from build123d import *

# Parameters (mm, degrees)
EXTRUDE_1_DEPTH     = 11
CUT_EXTRUDE_1_REACH = 15.892
SKETCH_2_R          = 1
CUT_EXTRUDE_2_REACH = 15.892
SKETCH_3_R          = 1


with BuildPart() as part:
    # 草图1 → 凸台-拉伸1 (new, symmetric)
    with BuildSketch(Plane(origin=(0, 0, 0), x_dir=(0, 0, -1), z_dir=(1, 0, 0))):
        Polygon((0, 0), (0, 6), (2, 6), (2, 2), (6, 2), (6, 0), align=None)
    extrude(amount=EXTRUDE_1_DEPTH, both=True)

    # 草图2 → 切除-拉伸1 (cut, up to next)
    with BuildSketch(Plane.XY, mode=Mode.PRIVATE) as cut_extrude_1_sk1:
        with Locations((-8.5, 4)):
            Circle(SKETCH_2_R)
    cut_extrude_1_tool1 = extrude(cut_extrude_1_sk1.sketch, amount=-CUT_EXTRUDE_1_REACH, mode=Mode.PRIVATE) & part.part
    # 草图2 → 切除-拉伸1 (cut, up to next)
    with BuildSketch(Plane.XY, mode=Mode.PRIVATE) as cut_extrude_1_sk2:
        with Locations((8.5, 4)):
            Circle(SKETCH_2_R)
    cut_extrude_1_tool2 = extrude(cut_extrude_1_sk2.sketch, amount=-CUT_EXTRUDE_1_REACH, mode=Mode.PRIVATE) & part.part
    add(cut_extrude_1_tool1.solids().sort_by_distance((-8.5, 4, 0))[0], mode=Mode.SUBTRACT)
    add(cut_extrude_1_tool2.solids().sort_by_distance((8.5, 4, 0))[0], mode=Mode.SUBTRACT)

    # 草图3 → 切除-拉伸2 (cut, up to next)
    with BuildSketch(Plane.XZ, mode=Mode.PRIVATE) as cut_extrude_2_sk1:
        with Locations(Location((-8.5, -4, 0), (0, 0, 270))):
            Circle(SKETCH_3_R)
    cut_extrude_2_tool1 = extrude(cut_extrude_2_sk1.sketch, amount=-CUT_EXTRUDE_2_REACH, mode=Mode.PRIVATE) & part.part
    # 草图3 → 切除-拉伸2 (cut, up to next)
    with BuildSketch(Plane.XZ, mode=Mode.PRIVATE) as cut_extrude_2_sk2:
        with Locations(Location((8.5, -4, 0), (0, 0, 270))):
            Circle(SKETCH_3_R)
    cut_extrude_2_tool2 = extrude(cut_extrude_2_sk2.sketch, amount=-CUT_EXTRUDE_2_REACH, mode=Mode.PRIVATE) & part.part
    add(cut_extrude_2_tool1.solids().sort_by_distance((-8.5, 0, -4))[0], mode=Mode.SUBTRACT)
    add(cut_extrude_2_tool2.solids().sort_by_distance((8.5, 0, -4))[0], mode=Mode.SUBTRACT)


solid = part.part
Build history of the part. All positions in model axes, mm. A direction names the side the tool comes from. Coordinates: 2 decimals unless noted, no trailing zeros. Order: outer loops, then holes, each group sorted by start corner. A loop starts at its lowest first (then second) coordinate and runs counter-clockwise, first axis right, second up. Notation, with made-up numbers: M 61.25,9 L 100.25,9 A22 cw 100.25,27 Z; hole C -18,75 d4. An arc over 180 degrees is marked long. One line per question, with ' | ' between items. Start each with the question number.
Q1. Two-plate mould, pull along Z, no slides. Class faces 3 (the face through (0, 1, -6)), 4 (the face through (0, 2, -4)), 5 (the face through (-7.51, 0.99, -3.87)), 6 (the face through (9.49, 0.99, -3.87)): +Z half, -Z half, draft (parallel to the pull), parting line (faces both ways), or undercut.
Q2. 3-axis set-ups, long thin cutter, end or side, ignore diameter. For faces 1 (the face through (0, 4, -2)), 2 (the face through (0, 3, 0)): which of +Z, -Z, +X, -X, +Y, -Y reach the whole face in a straight line?
Q3. Saw through at C-C (x = -8.5). List the corners of the cut face in (y, z), then the cut area to 3 significant figures.
Q4. Saw through at D-D (y = 1.4). List the corners of the cut face in (x, z).
Q5. Saw through at B-B (z = -4). List the corners of the cut face in (x, y).
Q6. Saw through at A-A (y = 4). List the corners of the cut face in (x, z).
Q7. Flat gauge pins, fed straight in: pin 1 Ø1.5 at (x, y) = (-0.5, 4) entering from -Z; pin 2 Ø3 at (x, z) = (8.5, -4) entering from +Y. Where does each tip first touch, or does it go through?
Q8. Probe L1, parallel to X at y = 3.95, z = -0.6; L2, parallel to Y at x = -8.5, z = -0.6; L3, parallel to Z at x = -5.75, y = 4.65. List the from-to ranges inside material, lowest first. Write a range as from..to.
Check values:
1) face 3: -Z half | face 4: draft | face 5: undercut | face 6: undercut
2) face 1: -Z, +X, -X, +Y | face 2: +Z, +X, -X, +Y, -Y
3) outline: M 0,-6 L 2,-6 L 2,-5 L 0,-5 Z; M 0,-3 L 2,-3 L 2,-2 L 3,-2 L 3,0 L 0,0 Z; M 5,-2 L 6,-2 L 6,0 L 5,0 Z | area: 12.0 mm2
4) outline: M -11,-6 L 11,-6 L 11,0 L -11,0 Z; hole C -8.5,-4 d2; hole C 8.5,-4 d2
5) outline: M -11,0 L -9.5,0 L -9.5,2 L -11,2 Z; M -7.5,0 L 7.5,0 L 7.5,2 L -7.5,2 Z; M 9.5,0 L 11,0 L 11,2 L 9.5,2 Z
6) outline: M -11,-2 L -9.5,-2 L -9.5,0 L -11,0 Z; M -7.5,-2 L 7.5,-2 L 7.5,0 L -7.5,0 Z; M 9.5,-2 L 11,-2 L 11,0 L 9.5,0 Z
7) pin 1: stops at z = -2 | pin 2: stops at y = 2
8) L1: x = -11..-9.5, -7.5..7.5, 9.5..11 | L2: y = 0..3, 5..6 | L3: z = -2..0
